from build123d import *

# Parameters (mm, degrees)
BOSS_EXTRUDE2_DEPTH = 50
SKETCH4_R           = 84
CUT_EXTRUDE1_DEPTH  = 40
SKETCH5_R           = 66
CUT_EXTRUDE2_DEPTH  = 40
SKETCH6_R           = 56
BOSS_EXTRUDE3_DEPTH = 20
SKETCH7_R           = 31
BOSS_EXTRUDE4_DEPTH = 20
SKETCH8_R           = 53
BOSS_EXTRUDE5_DEPTH = 30
SKETCH9_R           = 81.118790055
BOSS_EXTRUDE6_DEPTH = 10
SKETCH10_R          = 77.994904394
BOSS_EXTRUDE7_DEPTH = 10


with BuildPart() as part:
    # Sketch3 → Boss-Extrude2 (new body)
    with BuildSketch(Plane(origin=(0, 0, 0), x_dir=(1, 0, 0), z_dir=(0, 1, 0))):
        with BuildLine():
            Line((-426.753144047, -312.117374747), (-99.343882551, 70.106841813))
            ThreePointArc((-99.343882551, 70.106841813), (-49.831824853, 107.501926674), (10.778427661, 120.777224017))
            Line((10.778427661, 120.777224017), (514.059836256, 120.777224017))
            ThreePointArc((514.059836256, 120.777224017), (594.059836256, 40.777224017), (514.059836256, -39.222775983))
            Line((514.059836256, -39.222775983), (196.291302455, -76.947554654))
            ThreePointArc((196.291302455, -76.947554654), (57.544015582, -119.983155247), (-56.683941268, -209.731951378))
            Line((-56.683941268, -209.731951378), (-268.224957691, -449.836925027))
            ThreePointArc((-268.224957691, -449.836925027), (-415.870847806, -459.691045091), (-426.753144047, -312.117374747))
        make_face()
    extrude(amount=BOSS_EXTRUDE2_DEPTH)

    # Sketch4 → Cut-Extrude1 (cut)
    with BuildSketch(Plane(origin=(0, 50, 0), x_dir=(1, 0, 0), z_dir=(0, 1, 0))):
        with Locations(Location((-347.009402169, -380.425029013, 0), (0, 0, 270))):
            Circle(SKETCH4_R)
    extrude(amount=-CUT_EXTRUDE1_DEPTH, mode=Mode.SUBTRACT)

    # Sketch5 → Cut-Extrude2 (cut)
    with BuildSketch(Plane(origin=(0, 50, 0), x_dir=(1, 0, 0), z_dir=(0, 1, 0))):
        with Locations(Location((514.059836256, 40.777224017, 0), (0, 0, 270))):
            Circle(SKETCH5_R)
    extrude(amount=-CUT_EXTRUDE2_DEPTH, mode=Mode.SUBTRACT)

    # Sketch6 → Boss-Extrude3 (add)
    with BuildSketch(Plane(origin=(0, 10, 0), x_dir=(1, 0, 0), z_dir=(0, 1, 0))):
        with Locations(Location((-347.009402169, -380.425029013, 0), (0, 0, 270))):
            Circle(SKETCH6_R)
    extrude(amount=BOSS_EXTRUDE3_DEPTH)

    # Sketch7 → Boss-Extrude4 (add)
    with BuildSketch(Plane(origin=(0, 30, 0), x_dir=(1, 0, 0), z_dir=(0, 1, 0))):
        with Locations(Location((-347.009402169, -380.425029013, 0), (0, 0, 270))):
            Circle(SKETCH7_R)
    extrude(amount=BOSS_EXTRUDE4_DEPTH)

    # Sketch8 → Boss-Extrude5 (add)
    with BuildSketch(Plane(origin=(0, 10, 0), x_dir=(1, 0, 0), z_dir=(0, 1, 0))):
        with Locations(Location((514.059836256, 40.777224017, 0), (0, 0, 270))):
            Circle(SKETCH8_R)
    extrude(amount=BOSS_EXTRUDE5_DEPTH)

    # Sketch9 → Boss-Extrude6 (add)
    with BuildSketch(Plane.XZ):
        with Locations(Location((0, 0, 0), (0, 0, 270))):
            Circle(SKETCH9_R)
    extrude(amount=BOSS_EXTRUDE6_DEPTH)

    # Sketch10 → Boss-Extrude7 (add)
    with BuildSketch(Plane(origin=(0, 50, 0), x_dir=(1, 0, 0), z_dir=(0, 1, 0))):
        with Locations(Location((0, 0, 0), (0, 0, 270))):
            Circle(SKETCH10_R)
    extrude(amount=BOSS_EXTRUDE7_DEPTH)


solid = part.part
Design review of the part built by this model. Coordinates are the model's own, in mm. A direction names the side the tool comes from. Round coordinates to 2 decimals unless told otherwise and drop trailing zeros. Write each loop counter-clockwise with the first axis right and the second up, starting at its lowest first coordinate (ties: lowest second). Pieces come first, ordered by that corner, then holes. Notation, with made-up numbers: (64.5, 50.5) - (85.5, 50.5) arc R14 ccw to (85.5, 72.5) - close; hole circle Ø6 at (30, 79.25). An arc over 180 degrees is marked (long way). Use a Markdown table: item, result. Add a question column.
1. We need section D-D (x = -244). State the section outline as (y, z) points, then the cut area to 3 significant figures.
2. Clearance check with flat-ended pins moving along their axes: pin 1 (1 mm diameter, centred on x = -12, y = 22.5, fed in from +Z); pin 2 (10 mm diameter, centred on x = -240, y = 33.5, fed in from +Z); pin 3 (5 mm diameter, centred on x = 295, y = 32.5, fed in from +Z). State where each tip first meets the part, or that it passes through.
3. We need section A-A (z = 365.5). State the section outline as (x, y) points, then the cut area to 3 significant figures.
4. We need section C-C (z = -6). State the section outline as (x, y) points, then the cut area to 3 significant figures.
5. We need section B-B (x = 0). State the section outline as (y, z) points, then the cut area to 3 significant figures.
6. Wall thickness on probe 1 along X at (y, z) = (24, -2); probe 2 along X at (y, z) = (38.5, 398.5); probe 3 along Y at (x, z) = (74.5, 72.5): over which ranges is each line inside the solid? List them lowest first.
7. Mouldability with a two-part tool opening along X and no side actions: class faces 4 (the face through (-414.12, 24.65, 461.18)), 5 (the face through (-377.27, 39.86, 373.7)), 6 (the face through (-160.97, 24.65, 328.1)) as +X half, -X half, draft (parallel to the pull), parting line (faces both ways), or undercut.
8. For faces 1 (the face through (1, 60, -1)), 2 (the face through (-371, 30, 405)), 3 (the face through (-49.36, -4.93, 64.373)), list the 3-axis set-ups (+Z, -Z, +X, -X, +Y, -Y) from which the entire face can be reached by the end or side of a thin tool; tool diameter is ignored.
Output:
| question | item | result |
|---|---|---|
| 1 | outline | (0, 98.77) - (50, 98.77) - (50, 422.34) - (0, 422.34) - close |
| 1 | area | 16,200 mm2 |
| 2 | pin 1 | stops at z = 166.76 |
| 2 | pin 2 | stops at z = 423.48 |
| 2 | pin 3 | stops at z = 65.53 |
| 3 | outline | (-450.94, 0) - (-193.92, 0) - (-193.92, 50) - (-264.35, 50) - (-264.35, 10) - (-293.03, 10) - (-293.03, 30) - (-319.84, 30) - (-319.84, 50) - (-374.18, 50) - (-374.18, 30) - (-400.98, 30) - (-400.98, 10) - (-429.67, 10) - (-429.67, 50) - (-450.94, 50) - close |
| 3 | area | 9,480 mm2 |
| 4 | outline | (-154.26, 0) - (-80.9, 0) - (-80.9, -10) - (80.9, -10) - (80.9, 0) - (586.11, 0) - (586.11, 50) - (570.15, 50) - (570.15, 10) - (554.05, 10) - (554.05, 40) - (474.07, 40) - (474.07, 10) - (457.97, 10) - (457.97, 50) - (77.76, 50) - (77.76, 60) - (-77.76, 60) - (-77.76, 50) - (-154.26, 50) - close |
| 4 | area | 38,100 mm2 |
| 5 | outline | (-10, -81.12) - (0, -81.12) - (0, -120.38) - (50, -120.38) - (50, -77.99) - (60, -77.99) - (60, 77.99) - (50, 77.99) - (50, 156.77) - (0, 156.77) - (0, 81.12) - (-10, 81.12) - close |
| 5 | area | 17,000 mm2 |
| 6 | probe 1 | x = -157.68 to 460.65, 477.93 to 550.19, 567.47 to 584.03 |
| 6 | probe 2 | x = -450.44 to -429.04, -372.19 to -321.82, -264.98 to -223 |
| 6 | probe 3 | y = 0 to 50 |
| 7 | face 4 | parting line |
| 7 | face 5 | undercut |
| 7 | face 6 | +X half |
| 8 | face 1 | +Z, -Z, +X, -X, +Y |
| 8 | face 2 | +Y |
| 8 | face 3 | -Y |
